```python
from build123d import *

# Parameters (mm, degrees)
F1_DEPTH = 3
F2_R     = 1.5
F3_DEPTH = 25
F5_DEPTH = 3


with BuildPart() as f1:
    # F0 (on Front) → F1 (new body)
    with BuildSketch(Plane.XZ):
        with BuildLine():
            Line((-75, -60), (75, -60))
            ThreePointArc((75, -60), (78.535534, -58.535534), (80, -55))
            Line((80, -55), (80, 55))
            ThreePointArc((80, 55), (78.535534, 58.535534), (75, 60))
            Line((75, 60), (-75, 60))
            ThreePointArc((-75, 60), (-78.535534, 58.535534), (-80, 55))
            Line((-80, 55), (-80, -55))
            ThreePointArc((-80, -55), (-78.535534, -58.535534), (-75, -60))
        make_face()
    extrude(amount=F1_DEPTH)

    # F2 (on Front) → F3 (cut)
    with BuildSketch(Plane.XZ):
        with Locations((-75, 55)):
            Circle(F2_R)
        with Locations((75, 55)):
            Circle(F2_R)
        with Locations((75, -55)):
            Circle(F2_R)
        with Locations((-75, -55)):
            Circle(F2_R)
    extrude(amount=F3_DEPTH, mode=Mode.SUBTRACT)

    # F4 (on face) → F5 (cut)
    with BuildSketch(Plane.XZ.offset(3)):
        with BuildLine():
            ThreePointArc((72.5, 47.5), (71.035534, 51.035534), (67.5, 52.5))
            Line((67.5, 52.5), (-67.5, 52.5))
            ThreePointArc((-67.5, 52.5), (-71.035534, 51.035534), (-72.5, 47.5))
            Line((-72.5, 47.5), (-72.5, -47.5))
            ThreePointArc((-72.5, -47.5), (-71.035534, -51.035534), (-67.5, -52.5))
            Line((-67.5, -52.5), (67.5, -52.5))
            ThreePointArc((67.5, -52.5), (71.035534, -51.035534), (72.5, -47.5))
            Line((72.5, -47.5), (72.5, 47.5))
        make_face()
    extrude(amount=-F5_DEPTH, mode=Mode.SUBTRACT)


solid = f1.part
```
Geometry: final body of the model. Coordinates: model frame, mm. A direction names the side the tool comes from. Coordinates: 2 decimals unless noted, no trailing zeros. Order: outer loops, then holes, each group sorted by start corner. A loop starts at its lowest first (then second) coordinate and runs counter-clockwise, first axis right, second up. Notation, with made-up numbers: M 54,49 L 93,49 A16 cw 93,68 Z; hole C -22,8.25 d8. An arc over 180 degrees is marked long. Answer in a Markdown table with one row per item. Add a question column.
Q1. Section query B-B on y = -1.3. Return the cut outline in (x, z), and give its area (3 significant figures).
Q2. Contact query for flat-ended pins moving along their axis: P1, Ø5, axis at x = -75, z = 55, coming from the -Y side; P2, Ø1.8, axis at x = 75, z = -55, coming from the +Y side. Output: stop coordinate, or through.
Q3. Section query C-C on z = -36. Return the cut outline in (x, y).
Q4. Line query: L1, parallel to X at y = -2.15, z = 55; L2, parallel to Z at x = 75, y = -1.3; L3, parallel to Z at x = 20, y = -0.8. Output: solid intervals per line, ascending.
Q5. Reachability of faces 1 (the cylindrical face through (-78, -1, 59)), 2 (the cylindrical face through (71.07, -1.52, 51)) from +Z, -Z, +X, -X, +Y, -Y: full face, straight path, thin tool, end or side. Return the list, or none.
Q6. Section query A-A on x = 63. Return the cut outline in (y, z), and give its area (3 significant figures).
Q7. Mould query, pull axis Z, two halves, no side actions, for faces 3 (the cylindrical face through (78, -1, -59)), 4 (the cylindrical face through (-71.07, -1.52, -51)), 5 (the flat face through (-6, 0, -53)). Classes: released by +Z, released by -Z, zero draft, split by the parting line, or undercut.
Completed:
| question | item | result |
|---|---|---|
| 1 | outline | M -80,-55 A5 ccw -75,-60 L 75,-60 A5 ccw 80,-55 L 80,55 A5 ccw 75,60 L -75,60 A5 ccw -80,55 Z; hole C -75,-55 d3; hole C -75,55 d3; hole M -72.5,-47.5 A5 ccw -67.5,-52.5 L 67.5,-52.5 A5 ccw 72.5,-47.5 L 72.5,47.5 A5 ccw 67.5,52.5 L -67.5,52.5 A5 ccw -72.5,47.5 Z; hole C 75,-55 d3; hole C 75,55 d3 |
| 1 | area | 3,950 mm2 |
| 2 | P1 | stops at y = -3 |
| 2 | P2 | passes through |
| 3 | outline | M -80,-3 L -72.5,-3 L -72.5,0 L -80,0 Z; M 72.5,-3 L 80,-3 L 80,0 L 72.5,0 Z |
| 4 | L1 | x = -80 to -76.5, -73.5 to 73.5, 76.5 to 80 |
| 4 | L2 | z = -60 to -56.5, -53.5 to 53.5, 56.5 to 60 |
| 4 | L3 | z = -60 to -52.5, 52.5 to 60 |
| 5 | face 1 | +Z, -X, +Y, -Y |
| 5 | face 2 | +Y, -Y |
| 6 | outline | M -3,-60 L 0,-60 L 0,-52.5 L -3,-52.5 Z; M -3,52.5 L 0,52.5 L 0,60 L -3,60 Z |
| 6 | area | 45.0 mm2 |
| 7 | face 3 | released by -Z |
| 7 | face 4 | undercut |
| 7 | face 5 | zero draft |
